Input: part model. Units: mm. Frame: model coordinates. A direction names the side the tool comes from. Round coordinates to 2 decimals unless told otherwise and drop trailing zeros. Loops run counter-clockwise (first coordinate to the right, second up) from the corner with the lowest first, then second, coordinate; pieces in that order, holes last. Notation, with made-up numbers: (-1.75, 47) -> (4.25, 47) arc R23 ccw to (4.25, 78) -> close; hole circle Ø10 at (24, 67). An arc over 180 degrees is marked (long way). Answer in a Markdown table with one row per item. Add a question column.
Q1. Ray query, L1, parallel to X at y = 10.5, z = -7 (3 decimals); L2, parallel to Y at x = -3.5, z = 10.25; L3, parallel to Z at x = -8.75, y = -5.5. Return the intervals inside material, ascending. Write a range as from..to.
Q2. Section D-D, the plane x = -6. Output: boundary loops of the cut face in (y, z).
Q3. Section C-C, the plane y = -5. Output: boundary loops of the cut face in (x, z).
Q4. Pin query (flat end, axial travel): pin 1 (12 mm diameter, centred on y = 17.5, z = 7.5, fed in from +X) (3 decimals); pin 2 (8 mm diameter, centred on x = 8, z = -7.5, fed in from +Y) (3 decimals); pin 3 (10 mm diameter, centred on y = 9.5, z = 5.5, fed in from +X); pin 4 (5.5 mm diameter, centred on y = 13.35, z = 0, fed in from +X). Return the tip coordinate at first contact, or that it passes through.
Q5. Mould query, pull axis Z, two halves, no side actions, for faces 5 (the face through (0.151, 20.654, 3.761)), 6 (the face through (6.518, 16.347, -0.132)), 7 (the face through (10.8, -8, -3)). Classes: pulls with the +Z half, pulls with the -Z half, needs draft (parallel to the pull), parting line crosses it, or undercut.
Q6. Section B-B, the plane z = -7.5. Output: boundary loops of the cut face in (x, y) (3 decimals).
Q7. Section A-A, the plane x = 8.5. Output: boundary loops of the cut face in (y, z).
Q8. Reachability of faces 1 (the face through (3.35, 13, 0)), 2 (the face through (0, -17, 11.7)), 3 (the face through (0, -5, 5.1)), 4 (the face through (9.775, 13, -4)) from +Z, -Z, +X, -X, +Y, -Y: full face, straight path, thin tool, end or side. Return the list, or none.
```python
from build123d import *

# Parameters (mm, degrees)
SALIENTE_EXTRUIR1_DEPTH    = 10.8
CORTAR_EXTRUIR1_DEPTH      = 28.076558127
CORTAR_EXTRUIR1_DEPTH_BACK = 28.076558127
CROQUIS4_W                 = 1.025
CROQUIS4_H                 = 17.1
CORTAR_EXTRUIR2_DEPTH      = 33.246404838
CORTAR_EXTRUIR2_DEPTH_BACK = 6.425
CROQUIS5_R                 = 3


with BuildPart() as part:
    # Croquis3 → Saliente-Extruir1 (new, symmetric)
    with BuildSketch(Plane(origin=(0, 0, 0), x_dir=(0, 0, -1), z_dir=(1, 0, 0))):
        with BuildLine():
            Line((11.7, 11.4), (11.7, -21.9))
            Line((11.7, -21.9), (-11.7, -21.9))
            Line((-11.7, -21.9), (-11.7, -12))
            Line((-11.7, -12), (-5.1, -12))
            Line((-5.1, -12), (-5.1, 3))
            ThreePointArc((-5.1, 3), (-3.495742753, 20.791485505), (11.7, 11.4))
        make_face()
    extrude(amount=SALIENTE_EXTRUIR1_DEPTH, both=True)

    # Croquis4 → Cortar-Extruir1 (cut, two sides: drawn at the far end of the back side and taken through both)
    with BuildSketch(Plane.XY.offset(-CORTAR_EXTRUIR1_DEPTH_BACK)):
        with Locations((10.2875, 13.35)):
            Rectangle(CROQUIS4_W, CROQUIS4_H)
    extrude(amount=CORTAR_EXTRUIR1_DEPTH + CORTAR_EXTRUIR1_DEPTH_BACK, mode=Mode.SUBTRACT)

    # Croquis5 → Cortar-Extruir2 (cut, two sides: drawn at the far end of the back side and taken through both)
    with BuildSketch(Plane(origin=(9.775, 0, 0), x_dir=(0, 0, -1), z_dir=(1, 0, 0)).offset(-CORTAR_EXTRUIR2_DEPTH_BACK)):
        with Locations(Location((0, 13.35, 0), (0, 0, 270))):
            Circle(CROQUIS5_R)
    extrude(amount=CORTAR_EXTRUIR2_DEPTH + CORTAR_EXTRUIR2_DEPTH_BACK, mode=Mode.SUBTRACT)


solid = part.part
```
Answer block:
| question | item | result |
|---|---|---|
| 1 | L1 | -10.8..9.775 |
| 1 | L2 | -21.9..-12 |
| 1 | L3 | -11.7..5.1 |
| 2 | outline | (-21.9, -11.7) -> (11.4, -11.7) arc R10.5 ccw (long way) to (3, 5.1) -> (-12, 5.1) -> (-12, 11.7) -> (-21.9, 11.7) -> close |
| 3 | outline | (-10.8, -11.7) -> (10.8, -11.7) -> (10.8, 5.1) -> (-10.8, 5.1) -> close |
| 4 | pin 1 | x = 9.775 |
| 4 | pin 2 | y = 21.645 |
| 4 | pin 3 | x = 10.8 |
| 4 | pin 4 | x = 3.35 |
| 5 | face 5 | parting line crosses it |
| 5 | face 6 | undercut |
| 5 | face 7 | needs draft |
| 6 | outline | (-10.8, -21.9) -> (10.8, -21.9) -> (10.8, 4.8) -> (9.775, 4.8) -> (9.775, 19.8) -> (-10.8, 19.8) -> close |
| 7 | outline | (-21.9, -11.7) -> (11.4, -11.7) arc R10.5 ccw (long way) to (3, 5.1) -> (-12, 5.1) -> (-12, 11.7) -> (-21.9, 11.7) -> close; hole circle Ø6 at (13.35, 0) |
| 8 | face 1 | +X |
| 8 | face 2 | +Z, +X, -X, +Y, -Y |
| 8 | face 3 | +Z, +X, -X |
| 8 | face 4 | +Z, -Z, +X, +Y |
